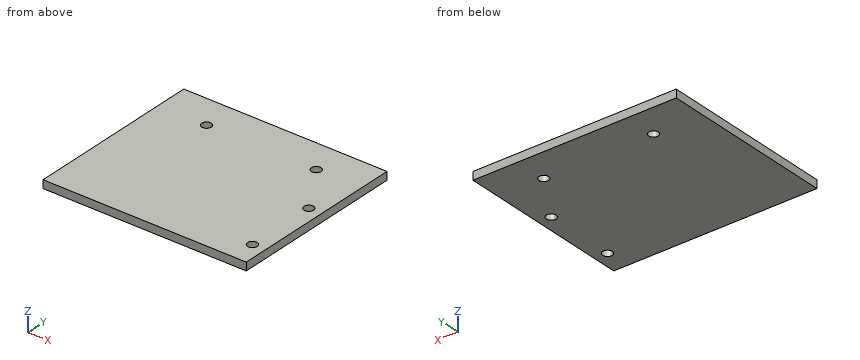
from build123d import *

# Parameters (mm, degrees)
SKETCH1_W           = 163
SKETCH1_H           = 150
BOSS_EXTRUDE1_DEPTH = 2.5
SKETCH3_R           = 1.5
CUT_EXTRUDE1_DEPTH  = 2.5
SKETCH4_W           = 4
SKETCH4_H           = 22
CUT_EXTRUDE2_DEPTH  = 111.785829419
SKETCH5_R           = 1.1
CUT_EXTRUDE3_DEPTH  = 111.785829419
CUT_EXTRUDE4_START  = -10
SKETCH6_W           = 4
SKETCH6_H           = 22
SKETCH6_R           = 1.5
SKETCH6_R_2         = 1.1
CUT_EXTRUDE4_DEPTH  = 10


with BuildPart() as part:
    # Sketch1 → Boss-Extrude1 (new body)
    with BuildSketch(Plane.XY):
        Rectangle(SKETCH1_W, SKETCH1_H)
    extrude(amount=BOSS_EXTRUDE1_DEPTH)

    # Sketch3 → Cut-Extrude1 (cut)
    with BuildSketch(Plane.XY.offset(2.5)):
        with Locations((-67.5, -30)):
            Circle(SKETCH3_R)
        with Locations((-33.5, -30)):
            Circle(SKETCH3_R)
        with Locations((-77.5, -45.5)):
            Circle(SKETCH3_R)
        with Locations((-77.5, -67.5)):
            Circle(SKETCH3_R)
    cut_extrude1 = extrude(amount=-CUT_EXTRUDE1_DEPTH, mode=Mode.SUBTRACT)

    # Mirror1: Cut-Extrude1 across plane
    add(cut_extrude1.mirror(Plane(origin=(0, 0, 0), x_dir=(0, 0, 1), z_dir=(1, 0, 0))), mode=Mode.SUBTRACT)

    # Sketch4 → Cut-Extrude2 (cut, through all)
    with BuildSketch(Plane.XY.offset(2.5)):
        with Locations((32.5, -7.5)):
            Rectangle(SKETCH4_W, SKETCH4_H)
        with Locations((-32.5, 27.5)):
            Rectangle(SKETCH4_W, SKETCH4_H)
        with Locations((-32.5, -7.5)):
            Rectangle(SKETCH4_W, SKETCH4_H)
        with Locations((32.5, 27.5)):
            Rectangle(SKETCH4_W, SKETCH4_H)
    extrude(amount=-CUT_EXTRUDE2_DEPTH, mode=Mode.SUBTRACT)

    # Sketch5 → Cut-Extrude3 (cut, through all)
    with BuildSketch(Plane.XY.offset(2.5)):
        with Locations((-28, 70)):
            Circle(SKETCH5_R)
        with Locations((28, 70)):
            Circle(SKETCH5_R)
    extrude(amount=-CUT_EXTRUDE3_DEPTH, mode=Mode.SUBTRACT)

    # Sketch6 → Cut-Extrude4 (cut)
    with BuildSketch(Plane(origin=(0, 0, 0), x_dir=(-1, 0, 0), z_dir=(0, 0, -1)).offset(CUT_EXTRUDE4_START)):
        Polygon((-18.5, -20), (-18.5, -75), (81.5, -75), (81.5, 75), (-81.5, 75), (-81.5, -20), align=None)
        with Locations((-32.5, -7.5)):
            Rectangle(SKETCH6_W, SKETCH6_H, mode=Mode.SUBTRACT)
        with Locations((77.5, -67.5)):
            Circle(SKETCH6_R, mode=Mode.SUBTRACT)
        with Locations((77.5, -45.5)):
            Circle(SKETCH6_R, mode=Mode.SUBTRACT)
        with Locations((33.5, -30)):
            Circle(SKETCH6_R, mode=Mode.SUBTRACT)
        with Locations((32.5, -7.5)):
            Rectangle(SKETCH6_W, SKETCH6_H, mode=Mode.SUBTRACT)
        with Locations((67.5, -30)):
            Circle(SKETCH6_R, mode=Mode.SUBTRACT)
        with Locations((-32.5, 27.5)):
            Rectangle(SKETCH6_W, SKETCH6_H, mode=Mode.SUBTRACT)
        with Locations((-28, 70)):
            Circle(SKETCH6_R_2, mode=Mode.SUBTRACT)
        with Locations((32.5, 27.5)):
            Rectangle(SKETCH6_W, SKETCH6_H, mode=Mode.SUBTRACT)
        with Locations((28, 70)):
            Circle(SKETCH6_R_2, mode=Mode.SUBTRACT)
    extrude(amount=CUT_EXTRUDE4_DEPTH, mode=Mode.SUBTRACT)


solid = part.part
Build history of the part. All positions in model axes, mm. Give positions to 0.01 mm unless a question says otherwise; leave off trailing zeros. Order: outer loops, then holes, each group sorted by start corner. A loop starts at its lowest first (then second) coordinate and runs counter-clockwise, first axis right, second up. Notation, with made-up numbers: M 21.5,35 L 73.5,35 A23 cw 73.5,61 Z; hole C 80.25,63 d8. An arc over 180 degrees is marked long. Use one line per item in the form item = value.
1) Saw through at A-A (x = 77.5). Give the cut face in (y, z).
Calculated:
outline = M -75,0 L -69,0 L -69,2.5 L -75,2.5 Z; M -66,0 L -47,0 L -47,2.5 L -66,2.5 Z; M -44,0 L -20,0 L -20,2.5 L -44,2.5 Z
2) Saw through at D-D (y = -45.5). Give the cut face in (x, z).
Calculated:
outline = M 18.5,0 L 76,0 L 76,2.5 L 18.5,2.5 Z; M 79,0 L 81.5,0 L 81.5,2.5 L 79,2.5 Z
3) Saw through at C-C (x = 33.5). Give the cut face in (y, z), plus the area to 3 significant figures.
Calculated:
outline = M -75,0 L -31.5,0 L -31.5,2.5 L -75,2.5 Z; M -28.5,0 L -20,0 L -20,2.5 L -28.5,2.5 Z
area = 130 mm2
4) Saw through at B-B (y = -30). Give the cut face in (x, z).
Calculated:
outline = M 18.5,0 L 32,0 L 32,2.5 L 18.5,2.5 Z; M 35,0 L 66,0 L 66,2.5 L 35,2.5 Z; M 69,0 L 81.5,0 L 81.5,2.5 L 69,2.5 Z
5) Probe probe 1 along Y at (x, z) = (77.5, 1); probe 2 along X at (y, z) = (-67.5, 1.95); probe 3 along X at (y, z) = (-31, 1.7). List the from-to ranges inside material, lowest first.
Calculated:
probe_1 = -75 to -69, -66 to -47, -44 to -20
probe_2 = 18.5 to 76, 79 to 81.5
probe_3 = 18.5 to 32.38, 34.62 to 66.38, 68.62 to 81.5
